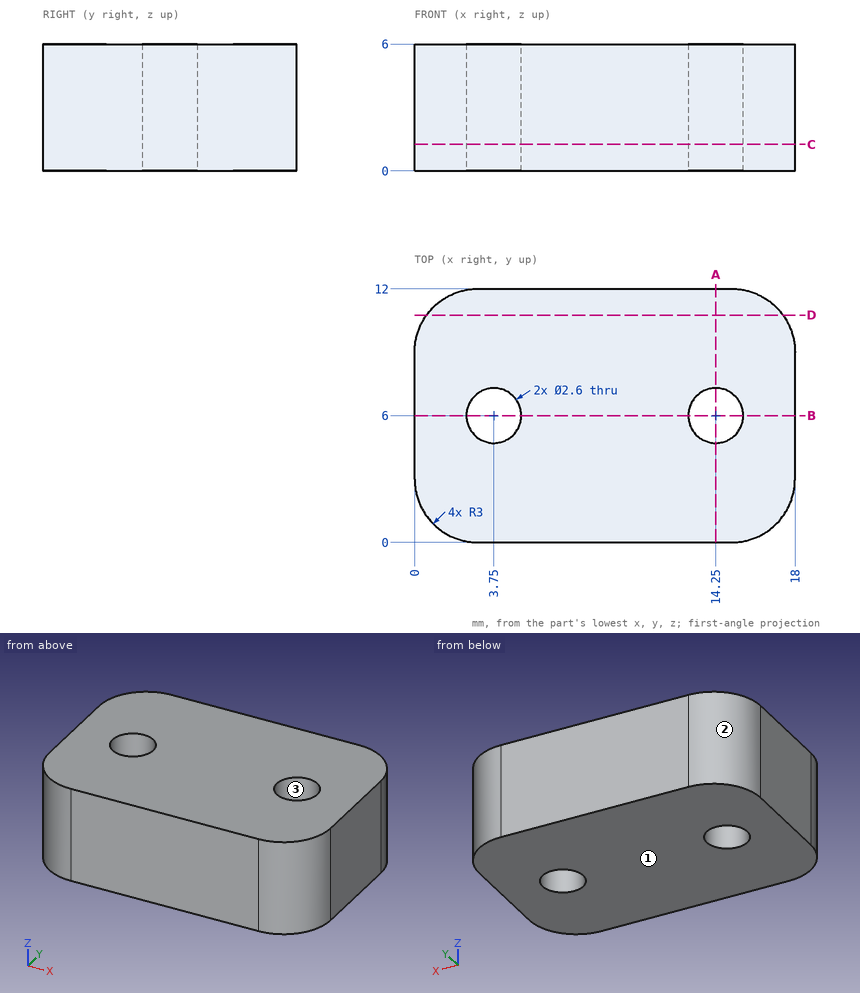
Verification items for this drawing (mm, ordinates from the low corner). Give positions to 0.01 mm unless a question says otherwise; leave off trailing zeros. Write each loop counter-clockwise with the first axis right and the second up, starting at its lowest first coordinate (ties: lowest second). Pieces come first, ordered by that corner, then holes.
1) Material ranges on L1, parallel to Y at x = 14.25, z = 2.7; L2, parallel to X at y = 6.25, z = 5.6; L3, parallel to X at y = 9.5, z = 4.85, recorded low to high.
2) Release check for a two-part mould opening along Y. For the marked faces 1, 2 and 3 record: pulls with the +Y half, pulls with the -Y half, needs draft (parallel to the pull), parting line crosses it, or undercut.
3) Section check C-C, the plane z = 1.25. Record the boundary of the cut face in (x, y), and give its area (3 significant figures).
4) Section check D-D, the plane y = 10.75. Record the boundary of the cut face in (x, z).
5) Section check B-B, the plane y = 6. Record the boundary of the cut face in (x, z).
6) Section check A-A, the plane x = 14.25. Record the boundary of the cut face in (y, z), and give its area (3 significant figures).
Computed:
1. L1: y = 0 to 4.7, 7.3 to 12
1. L2: x = 0 to 2.47, 5.03 to 12.97, 15.53 to 18
1. L3: x = 0.04 to 17.96
2. face 1: needs draft
2. face 2: pulls with the +Y half
2. face 3: undercut
3. outline: (0, 3) arc R3 ccw to (3, 0) - (15, 0) arc R3 ccw to (18, 3) - (18, 9) arc R3 ccw to (15, 12) - (3, 12) arc R3 ccw to (0, 9) - close; hole circle Ø2.6 at (3.75, 6); hole circle Ø2.6 at (14.25, 6)
3. area: 198 mm2
4. outline: (0.56, 0) - (17.44, 0) - (17.44, 6) - (0.56, 6) - close
5. outline: (0, 0) - (2.45, 0) - (2.45, 6) - (0, 6) - close; (5.05, 0) - (12.95, 0) - (12.95, 6) - (5.05, 6) - close; (15.55, 0) - (18, 0) - (18, 6) - (15.55, 6) - close
6. outline: (0, 0) - (4.7, 0) - (4.7, 6) - (0, 6) - close; (7.3, 0) - (12, 0) - (12, 6) - (7.3, 6) - close
6. area: 56.4 mm2
